Source: CAD feature listing. Evaluate the final solid. Frame: model axes, mm. A direction names the side the tool comes from. Give positions to 0.01 mm unless a question says otherwise; leave off trailing zeros. Loops run counter-clockwise (first coordinate to the right, second up) from the corner with the lowest first, then second, coordinate; pieces in that order, holes last. Notation, with made-up numbers: (43, 40.5) -> (74, 40.5) arc R20 ccw to (74, 52.5) -> close; hole circle Ø7 at (-9, -16). An arc over 180 degrees is marked (long way). Return JSON: item names as keys, results as strings. Group by question number.
(1) Draft query along Z for faces 3 (the face through (0, 2, 6)), 4 (the face through (-61.455, 1.014, -31.015)). Return one class per face: released by +Z, released by -Z, zero draft, split by the parting line, or undercut.
(2) Access query for faces 1 (the face through (0, 0, 6)), 2 (the face through (-34.66, 0.99, -13.48)). Directions: +Z, -Z, +X, -X, +Y, -Y. A direction counts if a zero-diameter tool reaches every point of the face in a straight line with its end or side. Return the directions, or none.
(3) Cut plane C-C on x = -33. Return loops of the section in (y, z).
(4) Ray query, line 1 (X direction, y = 0.75, z = 7.5); line 2 (Z direction, x = 19, y = 0.85); line 3 (X direction, y = 0.4, z = -11). Return the intervals inside material, ascending. Write a range as from..to.
(5) Cut plane B-B on z = 33. Return loops of the section in (x, y).
(6) Pin query (flat end, axial travel): pin 1 (2 mm diameter, centred on x = -74.81, z = 57.75, fed in from -Y). Return the tip coordinate at first contact, or that it passes through.
(7) Cut plane D-D on y = 1.55. Give the number of separate pieces and of enclosed holes in the cut face, then the cut area to 3 significant figures.
(8) Cut plane A-A on x = 9.5. Return loops of the section in (y, z).
```python
from build123d import *

# Parameters (mm, degrees)
SKETCH1_W           = 170
SKETCH1_H           = 127
BOSS_EXTRUDE1_DEPTH = 2
FILLET1_R           = 5
FILLET2_R           = 3
SKETCH2_R           = 1.75
CUT_EXTRUDE1_DEPTH  = 3
FILLET3_R           = 5


with BuildPart() as part:
    # Sketch1 → Boss-Extrude1 (new body)
    with BuildSketch(Plane(origin=(0, 0, 0), x_dir=(1, 0, 0), z_dir=(0, 1, 0))):
        with Locations((0.791433892, -6.955632319)):
            Rectangle(SKETCH1_W, SKETCH1_H)
        Polygon((-54.546913293, 44.544367681), (56.129781077, 44.544367681), (0.791433892, 0.699369526), align=None, mode=Mode.SUBTRACT)
        Polygon((-64.208566108, 36.889365836), (-64.208566108, -50.800630474), (-8.870218923, -6.955632319), align=None, mode=Mode.SUBTRACT)
        Polygon((-54.546913293, -58.455632319), (56.129781077, -58.455632319), (0.791433892, -14.610634164), align=None, mode=Mode.SUBTRACT)
        Polygon((65.791433892, 36.889365836), (65.791433892, -50.800630474), (10.453086707, -6.955632319), align=None, mode=Mode.SUBTRACT)
    extrude(amount=BOSS_EXTRUDE1_DEPTH)

    # Fillet1
    fillet1_edges = [part.edges().sort_by_distance(p)[0] for p in [
        (0.791433892, 1, -0.699369526),
        (56.129781077, 1, -44.544367681),
        (-54.546913293, 1, -44.544367681),
        (10.453086707, 1, 6.955632319),
        (65.791433892, 1, 50.800630474),
        (65.791433892, 1, -36.889365836),
        (-8.870218923, 1, 6.955632319),
        (-64.208566108, 1, -36.889365836),
        (-64.208566108, 1, 50.800630474),
        (56.129781077, 1, 58.455632319),
        (0.791433892, 1, 14.610634164),
    ]]
    fillet(fillet1_edges, radius=FILLET1_R)

    # Fillet2
    fillet2_edges = [part.edges().sort_by_distance(p)[0] for p in [
        (-84.208566108, 1, -56.544367681),
        (85.791433892, 1, -56.544367681),
        (85.791433892, 1, 70.455632319),
        (-84.208566108, 1, 70.455632319),
    ]]
    fillet(fillet2_edges, radius=FILLET2_R)

    # Sketch2 → Cut-Extrude1 (cut)
    with BuildSketch(Plane(origin=(0, 2, 0), x_dir=(1, 0, 0), z_dir=(0, 1, 0))):
        with Locations(Location((-75.408566108, 43.844367681, 0), (0, 0, 270))):
            Circle(SKETCH2_R)
        with Locations(Location((76.39143389, 43.843581312, 0), (0, 0, 270))):
            Circle(SKETCH2_R)
        with Locations(Location((76.991433894, -57.754647019, 0), (0, 0, 270))):
            Circle(SKETCH2_R)
        with Locations(Location((-74.808566104, -57.75386065, 0), (0, 0, 270))):
            Circle(SKETCH2_R)
    extrude(amount=-CUT_EXTRUDE1_DEPTH, mode=Mode.SUBTRACT)

    # Fillet3
    fillet3_edges = [part.edges().sort_by_distance(p)[0] for p in [
        (-54.546913293, 1, 58.455632319),
    ]]
    fillet(fillet3_edges, radius=FILLET3_R)


solid = part.part
```
Answers:
{
 "1": {"face 3": "zero draft", "face 4": "undercut"},
 "2": {"face 1": "+Z, -Z, +X, -X, -Y", "face 2": "+Y, -Y"},
 "3": {"outline": "(0, -56.54) -> (2, -56.54) -> (2, -44.54) -> (0, -44.54) -> close; (0, -27.47) -> (2, -27.47) -> (2, -12.16) -> (0, -12.16) -> close; (0, 26.07) -> (2, 26.07) -> (2, 41.38) -> (0, 41.38) -> close; (0, 58.46) -> (2, 58.46) -> (2, 70.46) -> (0, 70.46) -> close"},
 "4": {"line 1": "-84.21..-64.21, -11.95..13.53, 65.79..85.79", "line 2": "-56.54..-44.54, -15.13..0.18, 13.73..29.04, 58.46..70.46", "line 3": "-84.21..-64.21, -31.53..-12.21, 13.79..33.12, 65.79..85.79"},
 "5": {"outline": "(-84.21, 0) -> (-64.21, 0) -> (-64.21, 2) -> (-84.21, 2) -> close; (-41.74, 0) -> (-22.42, 0) -> (-22.42, 2) -> (-41.74, 2) -> close; (24, 0) -> (43.32, 0) -> (43.32, 2) -> (24, 2) -> close; (65.79, 0) -> (85.79, 0) -> (85.79, 2) -> (65.79, 2) -> close"},
 "6": {"pin 1": "through"},
 "7": {"separate pieces": "1", "enclosed holes": "8", "area": "12,100 mm²"},
 "8": {"outline": "(0, -56.54) -> (2, -56.54) -> (2, -44.54) -> (0, -44.54) -> close; (0, -7.6) -> (2, -7.6) -> (2, 21.51) -> (0, 21.51) -> close; (0, 58.46) -> (2, 58.46) -> (2, 70.46) -> (0, 70.46) -> close"}
}
